Could you check a few things on this model? Use its own coordinates, in mm. A direction names the side the tool comes from. Round coordinates to 2 decimals unless told otherwise and drop trailing zeros. Loops run counter-clockwise (first coordinate to the right, second up) from the corner with the lowest first, then second, coordinate; pieces in that order, holes last. Notation, with made-up numbers: (69.25, 86.25) -> (110.25, 86.25) arc R24 cw to (110.25, 114.25) -> close; hole circle Ø8 at (72, -14). An arc over 180 degrees is marked (long way). One line per item, written item: value.
from build123d import *

# Parameters (mm, degrees)
F0_W      = 160
F0_H      = 284
F1_DEPTH  = 1
F2_W      = 160
F2_H      = 284
F2_W_2    = 158
F2_H_2    = 282
F3_DEPTH  = 24
F4_W      = 1.5
F4_H      = 1.5
F5_DEPTH  = 25.001
F6_R      = 6
F6_R_2    = 4
F7_DEPTH  = 25.001
F8_W      = 157
F8_H      = 1
F9_DEPTH  = 15
F10_R     = 3
F12_DEPTH = 1.001
F13_W     = 1
F13_H     = 8
F14_DEPTH = 5
F15_W     = 1
F15_H     = 3
F16_DEPTH = 6
F17_R     = 0.99999
F18_R     = 0.99999


# Not quite as in the source:
# - a fillet or chamfer is up to 0.001 mm smaller than in the source, because OpenCascade refuses the exact size


with BuildPart() as f1:
    # F0 (on Front) → F1 (new body)
    with BuildSketch(Plane.XZ):
        with Locations((80, 142)):
            Rectangle(F0_W, F0_H)
    extrude(amount=F1_DEPTH)

    # F2 (on face) → F3 (join)
    with BuildSketch(Plane(origin=(0, 0, 0), x_dir=(-1, 0, 0), z_dir=(0, 1, 0))):
        with Locations((-80, 142)):
            Rectangle(F2_W, F2_H)
        with Locations((-80, 142)):
            Rectangle(F2_W_2, F2_H_2, mode=Mode.SUBTRACT)
    extrude(amount=F3_DEPTH)

    # F4 (on face) → F5 (cut, through all)
    with BuildSketch(Plane.XZ.offset(1)):
        with Locations((0.75, 283.25)):
            Rectangle(F4_W, F4_H)
        with Locations((159.25, 283.25)):
            Rectangle(F4_W, F4_H)
        with Locations((159.25, 0.75)):
            Rectangle(F4_W, F4_H)
        with Locations((0.75, 0.75)):
            Rectangle(F4_W, F4_H)
    extrude(amount=-F5_DEPTH, mode=Mode.SUBTRACT)

    # F6 (on face) → F7 (cut, through all)
    with BuildSketch(Plane.XZ.offset(1)):
        with Locations((132.5, 124.5)):
            Circle(F6_R)
        with Locations((132.5, 109.5)):
            Circle(F6_R_2)
        with Locations((132.5, 94.5)):
            Circle(F6_R)
        with Locations((132.5, 79.5)):
            Circle(F6_R)
        with Locations((132.5, 64.5)):
            Circle(F6_R)
        with Locations((132.5, 49.5)):
            Circle(F6_R)
    extrude(amount=-F7_DEPTH, mode=Mode.SUBTRACT)

    # F8 (on face) → F9 (join)
    with BuildSketch(Plane(origin=(0, 0, 0), x_dir=(1, 0, 0), z_dir=(0, 0, -1))):
        with Locations((80, -23.5)):
            Rectangle(F8_W, F8_H)
    extrude(amount=F9_DEPTH)

    # F10
    f10_edges = [f1.edges().sort_by_distance(p)[0] for p in [
        (1.5, 23.5, -15),
        (158.5, 23.5, -15),
    ]]
    fillet(f10_edges, radius=F10_R)

    # F11 (on face) → F12 (cut, through all)
    with BuildSketch(Plane.XZ.offset(-23)):
        with BuildLine():
            ThreePointArc((16.3, -7.8), (14.5, -6), (12.7, -7.8))
            Line((12.7, -7.8), (12.7, -10.2))
            ThreePointArc((12.7, -10.2), (14.5, -12), (16.3, -10.2))
            Line((16.3, -10.2), (16.3, -7.8))
        make_face()
        with BuildLine():
            ThreePointArc((147.3, -7.8), (145.5, -6), (143.7, -7.8))
            Line((143.7, -7.8), (143.7, -10.2))
            ThreePointArc((143.7, -10.2), (145.5, -12), (147.3, -10.2))
            Line((147.3, -10.2), (147.3, -7.8))
        make_face()
    extrude(amount=-F12_DEPTH, mode=Mode.SUBTRACT)

    # F13 (on face) → F14 (join)
    with BuildSketch(Plane(origin=(0, 24, 0), x_dir=(-1, 0, 0), z_dir=(0, 1, 0))):
        with Locations((-159.5, 267.5)):
            Rectangle(F13_W, F13_H)
        with Locations((-0.5, 267.5)):
            Rectangle(F13_W, F13_H)
    extrude(amount=F14_DEPTH)

    # F15 (on face) → F16 (join)
    with BuildSketch(Plane(origin=(0, 0, 263.5), x_dir=(1, 0, 0), z_dir=(0, 0, -1))):
        with Locations((159.5, -27.5)):
            Rectangle(F15_W, F15_H)
        with Locations((0.5, -27.5)):
            Rectangle(F15_W, F15_H)
    extrude(amount=F16_DEPTH)

    # F17 (radius 1 in the source; OpenCascade refuses exactly that, so slightly less here)
    f17_edges = [f1.edges().sort_by_distance(p)[0] for p in [
        (0.5, 26, 263.5),
        (0.5, 26, 257.5),
        (0.5, 29, 257.5),
        (0.5, 24, 263.5),
        (0.5, 24, 271.5),
        (0.5, 29, 271.5),
    ]]
    fillet(f17_edges, radius=F17_R)

    # F18 (radius 1 in the source; OpenCascade refuses exactly that, so slightly less here)
    f18_edges = [f1.edges().sort_by_distance(p)[0] for p in [
        (159.5, 24, 271.5),
        (159.5, 29, 271.5),
        (159.5, 29, 257.5),
        (159.5, 24, 263.5),
        (159.5, 26, 257.5),
        (159.5, 26, 263.5),
    ]]
    fillet(f18_edges, radius=F18_R)


solid = f1.part
(1) For faces 1 (the face through (1, 14, 140)), 2 (the face through (79, -1, 144)), 3 (the face through (79, 23, -7)), 4 (the face through (79, 0, 144)), 5 (the face through (81, 12, 1)), which set-ups out of +Z, -Z, +X, -X, +Y, -Y let a thin tool reach every point of the face, with its end or its side?
Recorded:
face 1: +Z, -Z, +Y
face 2: +Z, -Z, +X, -X, -Y
face 3: -Z, +X, -X, -Y
face 4: +Y
face 5: +X, -X, +Y
(2) If we section it at C-C, the plane x = 132.5: Give the number of separate pieces and of enclosed holes in the cut face, then the cut area to 3 significant figures.
Recorded:
separate pieces: 7
enclosed holes: 0
area: 279 mm²
(3) If we section it at D-D, the plane z = 247: Please give me the cut outline in (x, y), then the cut area to 3 significant figures.
Recorded:
outline: (0, -1) -> (160, -1) -> (160, 24) -> (159, 24) -> (159, 0) -> (1, 0) -> (1, 24) -> (0, 24) -> close
area: 208 mm²
(4) I'm going to push flat-ended pins straight in: pin 1 Ø0.8 at (x, z) = (159.5, 111.5) entering from +Y; pin 2 Ø1.5 at (x, z) = (91, 238) entering from +Y; pin 3 Ø12 at (x, y) = (41.5, 16) entering from -Z. Where does each tip first touch, or does it pass through?
Recorded:
pin 1: y = 24
pin 2: y = 0
pin 3: z = 0
(5) If I drill on L1, parallel to X at y = 0.75, z = 6; L2, parallel to Z at x = 55, y = 20.5; L3, parallel to Y at x = 151.5, z = 194, over which ranges is the centre line in solid material (lowest first)?
Recorded:
L1: 0 to 1, 159 to 160
L2: 0 to 1, 283 to 284
L3: -1 to 0
(6) Thinking about a two-plate mould opening in X: for faces 6 (the face through (131.979, -0.507, 113.466)), 7 (the face through (81, 12, 283)), 8 (the face through (158.5, 15.3, 0.3)), which applies, released by +X, released by -X, zero draft, split by the parting line, or undercut?
Recorded:
face 6: undercut
face 7: zero draft
face 8: released by +X
(7) If we section it at A-A, the plane z = 49.5: Please give me the cut outline in (x, y).
Recorded:
outline: (0, -1) -> (126.5, -1) -> (126.5, 0) -> (1, 0) -> (1, 24) -> (0, 24) -> close; (138.5, -1) -> (160, -1) -> (160, 24) -> (159, 24) -> (159, 0) -> (138.5, 0) -> close
(8) If we section it at B-B, the plane y = 13.5: Please give me the cut outline in (x, z).
Recorded:
outline: (0, 1.5) -> (1, 1.5) -> (1, 282.5) -> (0, 282.5) -> close; (1.5, 0) -> (158.5, 0) -> (158.5, 1) -> (1.5, 1) -> close; (1.5, 283) -> (158.5, 283) -> (158.5, 284) -> (1.5, 284) -> close; (159, 1.5) -> (160, 1.5) -> (160, 282.5) -> (159, 282.5) -> close
